Geometry: see drawing. Coordinates: mm, zero at the bounding-box minimum. Coordinates: 2 decimals unless noted, no trailing zeros. Loops run counter-clockwise (first coordinate to the right, second up) from the corner with the lowest first, then second, coordinate; pieces in that order, holes last.
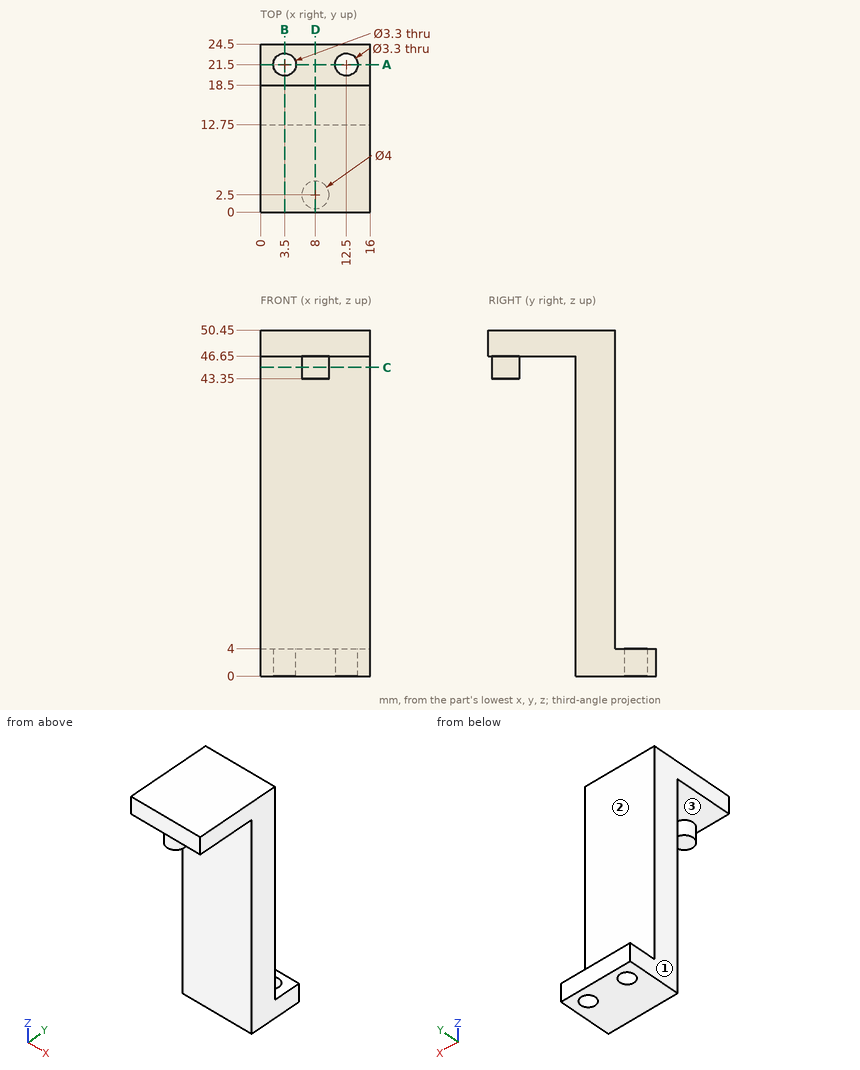
Item 1: Section query B-B (x = 3.5). Output: boundary loops of the cut face in (y, z).
Result:
outline: (0, 46.65) - (12.75, 46.65) - (12.75, 0) - (19.85, 0) - (19.85, 4) - (18.5, 4) - (18.5, 50.45) - (0, 50.45) - close; (23.15, 0) - (24.5, 0) - (24.5, 4) - (23.15, 4) - close
Item 2: Mould query, pull axis Y, two halves, no side actions, for the marked faces 1, 2 and 3. Classes: +Y half, -Y half, draft (parallel to the pull), parting line (faces both ways), or undercut.
Result:
face 1: draft
face 2: +Y half
face 3: undercut
Item 3: Section query C-C (z = 45). Output: boundary loops of the cut face in (x, y), then the cut area to 3 significant figures.
Result:
outline: (0, 12.75) - (16, 12.75) - (16, 18.5) - (0, 18.5) - close; circle Ø4 at (8, 2.5)
area: 105 mm2
Item 4: Section query D-D (x = 8). Output: boundary loops of the cut face in (y, z).
Result:
outline: (0, 46.65) - (0.5, 46.65) - (0.5, 43.35) - (4.5, 43.35) - (4.5, 46.65) - (12.75, 46.65) - (12.75, 0) - (24.5, 0) - (24.5, 4) - (18.5, 4) - (18.5, 50.45) - (0, 50.45) - close
Item 5: Contact query for flat-ended pins moving along their axis: P1, Ø2, axis at x = 9, y = 2.5, coming from the -Z side; P2, Ø5, axis at x = 11.5, z = 23, coming from the +Y side; P3, Ø1.5, axis at x = 4, y = 13.5, coming from the -Z side; P4, Ø2, axis at x = 12.5, y = 21.5, coming from the +Z side. Output: stop coordinate, or through.
Result:
P1: stops at z = 43.35
P2: stops at y = 18.5
P3: stops at z = 0
P4: passes through
Item 6: Line query: L1, parallel to X at y = 21.5, z = 2.6; L2, parallel to Y at x = 12.5, z = 1.6; L3, parallel to Y at x = 3, z = 17.5. Output: solid intervals per line, ascending.
Result:
L1: x = 0 to 1.85, 5.15 to 10.85, 14.15 to 16
L2: y = 12.75 to 19.85, 23.15 to 24.5
L3: y = 12.75 to 18.5
Item 7: Section query A-A (y = 21.5). Output: boundary loops of the cut face in (x, z).
Result:
outline: (0, 0) - (1.85, 0) - (1.85, 4) - (0, 4) - close; (5.15, 0) - (10.85, 0) - (10.85, 4) - (5.15, 4) - close; (14.15, 0) - (16, 0) - (16, 4) - (14.15, 4) - close
